The figure shows three views and two pictorial views of one solid part (mm, origin at its lowest corner). Answer the questions. Coordinates: 2 decimals unless noted, no trailing zeros. Loops run counter-clockwise (first coordinate to the right, second up) from the corner with the lowest first, then second, coordinate; pieces in that order, holes last. Notation, with made-up numbers: (61, -25.5) - (117, -25.5) arc R17 cw to (117, -21.5) - close; hole circle Ø8 at (-11.75, 42.5). An arc over 180 degrees is marked (long way). Return JSON: item names as keys, results as strings. Group by question number.
1. Section A-A (z = 34) is taken. Write down the section's boundary in (x, y).
2. Section B-B (x = 34.5) is taken. Write down the section's boundary in (y, z).
3. Section C-C (x = 5.5) is taken. Write down the section's boundary in (y, z).
4. Section D-D (y = 1.2) is taken. State how many separate pieces and enclosed holes the cut face has, and give its area (3 significant figures).
5. Find the intervals of material crossed by line 1 along Z through (x, y) = (144, 1.3); line 2 along X through (y, z) = (1.95, 42); line 3 along Z through (x, y) = (30, 1.6), in increasing order.
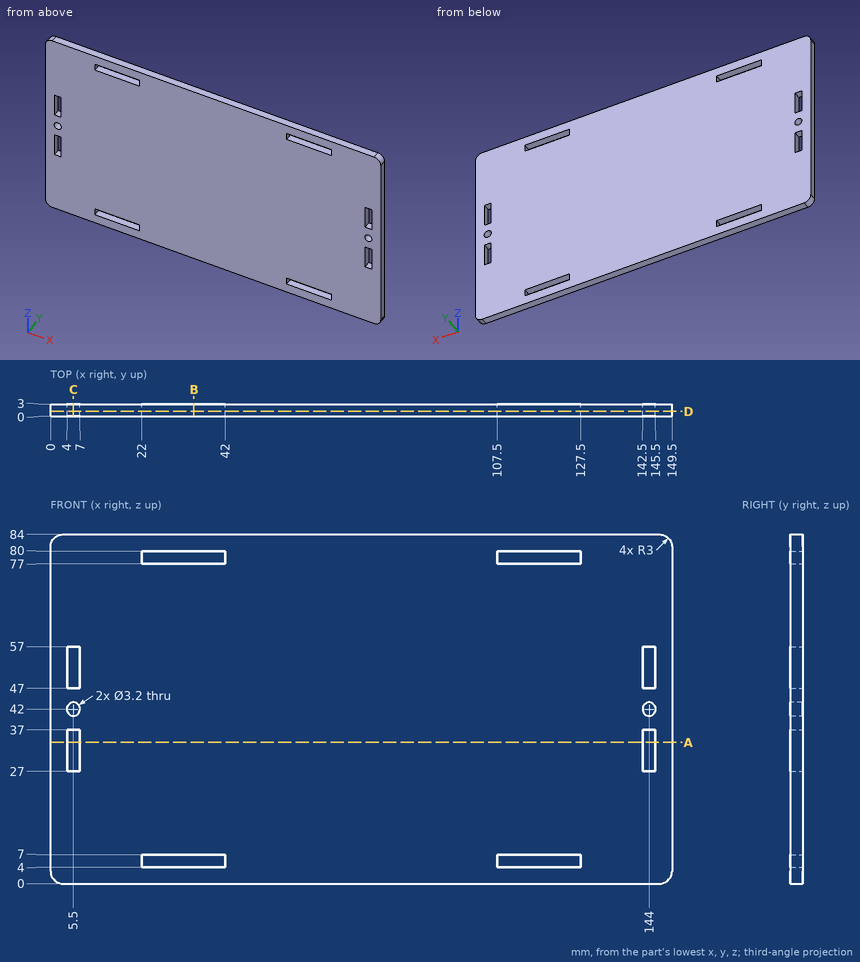
The answers:
{
 "1": {"outline": "(0, 0) - (4, 0) - (4, 3) - (0, 3) - close; (7, 0) - (142.5, 0) - (142.5, 3) - (7, 3) - close; (145.5, 0) - (149.5, 0) - (149.5, 3) - (145.5, 3) - close"},
 "2": {"outline": "(0, 0) - (3, 0) - (3, 4) - (0, 4) - close; (0, 7) - (3, 7) - (3, 77) - (0, 77) - close; (0, 80) - (3, 80) - (3, 84) - (0, 84) - close"},
 "3": {"outline": "(0, 0) - (3, 0) - (3, 27) - (0, 27) - close; (0, 37) - (3, 37) - (3, 40.4) - (0, 40.4) - close; (0, 43.6) - (3, 43.6) - (3, 47) - (0, 47) - close; (0, 57) - (3, 57) - (3, 84) - (0, 84) - close"},
 "4": {"separate pieces": "1", "enclosed holes": "10", "area": "12,200 mm2"},
 "5": {"line 1": "z = 0 to 27, 37 to 40.4, 43.6 to 47, 57 to 84", "line 2": "x = 0 to 3.9, 7.1 to 142.4, 145.6 to 149.5", "line 3": "z = 0 to 4, 7 to 77, 80 to 84"}
}
